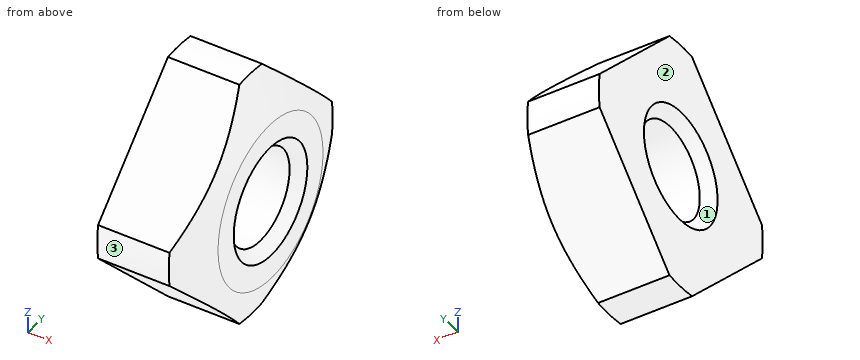
Autodesk Inventor part; units mm, degrees
ref_plane "IP1_XY" through (0, 0, 0) normal (1, 0, 0) x (0, 0, -1)
ref_plane "IP1_YZ" through (0, 0, 0) normal (0, 0, -1) x (0, 1, 0)
ref_plane "IP1_ZX" through (0, 0, 0) normal (0, 1, 0) x (1, 0, 0)
sketch "Sketch_2" plane through (0, 0, 0) normal (0, 0, 1) x (1, 0, 0)
  line L0 (3.2, 0) -> (0, 0)
  line L1 (0, 0) -> (0, 4.9497)
  line L2 (0, 4.9497) -> (2.287, 4.9497)
  line L3 (2.287, 4.9497) -> (3.2, 2.85)
  line L4 (3.2, 2.85) -> (3.2, 0)
  line L5 (3.2, 0) -> (0, 0)
revolve "Revolution1" add sketch "Sketch_2" angle 360 about axis through (3.2, 0, 0) along (1, 0, 0)
sketch "Skizze_2" plane through (0, 0, 0) normal (1, 0, 0) x (0, 1, 0)
  line L0 (14, 14) -> (-14, 14)
  line L1 (-14, 14) -> (-14, -14)
  line L2 (-14, -14) -> (14, -14)
  line L3 (14, -14) -> (14, 14)
  line L4 (0, 5.0205) -> (-5.0205, 0)
  line L5 (-5.0205, 0) -> (0, -5.0205)
  line L6 (0, -5.0205) -> (5.0205, 0)
  line L7 (5.0205, 0) -> (0, 5.0205)
extrude "Extrusion1" cut sketch "Skizze_2" along normal blind 3.2
sketch "Sketch_1" plane through (0, 0, 0) normal (0, 0, 1) x (1, 0, 0)
  line L0 (3.2, 0) -> (0, 0)
  line L1 (0, 0) -> (0, 2)
  line L2 (0, 2) -> (0.379, 1.621)
  line L3 (0.379, 1.621) -> (2.821, 1.621)
  line L4 (2.821, 1.621) -> (3.2, 2)
  line L5 (3.2, 2) -> (3.2, 0)
  line L6 (3.2, 0) -> (0, 0)
revolve "Revolution2" cut sketch "Sketch_1" angle 360 about axis through (3.2, 0, 0) along (1, 0, 0)
sketch "Sketch_3" plane through (0, 0, 0) normal (1, 0, 0) x (0, 1, 0)
  line L0 (7, 7) -> (-7, 7)
  line L1 (-7, 7) -> (-7, -7)
  line L2 (-7, -7) -> (7, -7)
  line L3 (7, -7) -> (7, 7)
  circle A0 centre (0, 0) radius 4.45
extrude "Extrusion2" cut sketch "Sketch_3" along normal blind 3.2
ref_plane "IP1_XY" through (0, 0, 0) normal (1, 0, 0) x (0, 0, -1)
ref_plane "IP1_YZ" through (0, 0, 0) normal (0, 0, -1) x (0, 1, 0)
ref_plane "IP1_ZX" through (0, 0, 0) normal (0, 1, 0) x (1, 0, 0)
ref_plane "IP2_XY" through (3.2, 0, 0) normal (1, 0, 0) x (0, 0, -1)
ref_plane "IP2_YZ" through (3.2, 0, 0) normal (0, 0, -1) x (0, 1, 0)
ref_plane "IP2_ZX" through (3.2, 0, 0) normal (0, 1, 0) x (1, 0, 0)
properties part number "DIN 557 - M4"
CAD build for the part. Positions are in the model's coordinates, mm. Face numbers are marked on the shaded views. Coordinates: 2 decimals unless noted, no trailing zeros. Order: outer loops, then holes, each group sorted by start corner. A loop starts at its lowest first (then second) coordinate and runs counter-clockwise, first axis right, second up. Notation, with made-up numbers: (-17, 66) - (1, 66) arc R16 ccw to (1, 92) - close; hole circle Ø4 at (40.25, -37). An arc over 180 degrees is marked (long way). Use a Markdown table: item, result. Add a question column.
(1) Saw through at C-C (x = 1.15). Give the cut face in (y, z), then the cut area to 3 significant figures.
(2) Drill centre lines: line 1 along Z through (x, y) = (1.5, 0); line 2 along Y through (x, z) = (1.35, 0.5). Where is each one in solid material? Low to high. Write a range as [from, to].
(3) Saw through at A-A (y = 0). Give the cut face in (x, z), then the cut area to 3 significant figures.
(4) Pull direction Y, two halves, no side cores. Call the marked faces 1, 2 and 3: +Y half, -Y half, draft (parallel to the pull), parting line (faces both ways), or undercut.
(5) Flat gauge pin, fed straight in: pin 1 (1 mm diameter, centred on x = 1, y = -1.5, fed in from +Z). Where does the tip first touch, or does it go through?
Solved:
| question | item | result |
|---|---|---|
| 1 | outline | (-4.41, -0.61) - (-0.61, -4.41) arc R4.45 ccw to (0.61, -4.41) - (4.41, -0.61) arc R4.45 ccw to (4.41, 0.61) - (0.61, 4.41) arc R4.45 ccw to (-0.61, 4.41) - (-4.41, 0.61) arc R4.45 ccw to start; hole circle Ø3.24 at (0, 0) |
| 1 | area | 40.8 mm² |
| 2 | line 1 | z = [-4.45, -1.62], [1.62, 4.45] |
| 2 | line 2 | y = [-4.42, -1.54], [1.54, 4.42] |
| 3 | outline | (0, -4.45) - (2.5, -4.45) - (3.2, -2.85) - (3.2, -2) - (2.82, -1.62) - (0.38, -1.62) - (0, -2) - close; (0, 2) - (0.38, 1.62) - (2.82, 1.62) - (3.2, 2) - (3.2, 2.85) - (2.5, 4.45) - (0, 4.45) - close |
| 3 | area | 16.7 mm² |
| 4 | face 1 | undercut |
| 4 | face 2 | draft |
| 4 | face 3 | -Y half |
| 5 | pin 1 | stops at z = 4.02 |
